Read the model definition and answer for the solid it produces. Units are mm, in the model's axes. Coordinates: 2 decimals unless noted, no trailing zeros. Order: outer loops, then holes, each group sorted by start corner. A loop starts at its lowest first (then second) coordinate and runs counter-clockwise, first axis right, second up. Notation, with made-up numbers: (28, 41.25) - (62, 41.25) arc R29 cw to (62, 65.25) - close; hole circle Ø4 at (-24.5, 75.25). An arc over 180 degrees is marked (long way). Write item = value, one per line.
from build123d import *

# Parameters (mm, degrees)
SKETCH1_W             = 80
SKETCH1_H             = 60
BOSS_EXTRUDE1_DEPTH   = 4.7625
M8_CLEARANCE_HOLE1_D  = 9
M6X1_0_TAPPED_HOLE2_D = 5
CHAMFER1_SIZE         = 1


with BuildPart() as part:
    # Sketch1 → Boss-Extrude1 (new, symmetric)
    with BuildSketch(Plane.XY):
        Rectangle(SKETCH1_W, SKETCH1_H)
    extrude(amount=BOSS_EXTRUDE1_DEPTH, both=True)

    # M8 Clearance Hole1 (through all)
    with Locations(Plane.XY.offset(4.7625)):
        with Locations((-30, 20), (30, 20), (30, -20), (-30, -20)):
            Hole(M8_CLEARANCE_HOLE1_D / 2)

    # M6x1.0 Tapped Hole2 (through all)
    with Locations(Plane.XY.offset(4.7625)):
        with Locations((-6.5, 23), (-6.5, -23)):
            Hole(M6X1_0_TAPPED_HOLE2_D / 2)

    # Chamfer1
    chamfer1_edges = [part.edges().sort_by_distance(p)[0] for p in [
        (-40, 30, 0),
        (40, 30, 0),
        (40, -30, 0),
        (-40, -30, 0),
    ]]
    chamfer(chamfer1_edges, length=CHAMFER1_SIZE)


solid = part.part
1) Determine the mould class of faces 1 (the face through (27.581, -16.206, -0.067)), 2 (the face through (-1, 30, 0)), 3 (the face through (-1, 0, 4.762)), 4 (the face through (-1, -30, 0)) for opening direction Y: pulls with the +Y half, pulls with the -Y half, needs draft (parallel to the pull), parting line crosses it, or undercut.
Returned:
face_1 = undercut
face_2 = pulls with the +Y half
face_3 = needs draft
face_4 = pulls with the -Y half
2) The part is cut by section B-B (z = 0.25). Determine the outline of the cut face in (x, y).
Returned:
outline = (-40, -29) - (-39, -30) - (39, -30) - (40, -29) - (40, 29) - (39, 30) - (-39, 30) - (-40, 29) - close; hole circle Ø9 at (-30, -20); hole circle Ø9 at (-30, 20); hole circle Ø5 at (-6.5, -23); hole circle Ø5 at (-6.5, 23); hole circle Ø9 at (30, -20); hole circle Ø9 at (30, 20)
3) The part is cut by section A-A (x = -30). Determine the outline of the cut face in (y, z).
Returned:
outline = (-30, -4.76) - (-24.5, -4.76) - (-24.5, 4.76) - (-30, 4.76) - close; (-15.5, -4.76) - (15.5, -4.76) - (15.5, 4.76) - (-15.5, 4.76) - close; (24.5, -4.76) - (30, -4.76) - (30, 4.76) - (24.5, 4.76) - close
4) Straight lines are drawn through the part: line 1 along Y through (x, z) = (-30, 0); line 2 along Y through (x, z) = (-6.5, -1.75); line 3 along X through (y, z) = (24, -1.5). For each, find the intervals that lie inside material, in ascending order. Write a range as from..to.
Returned:
line_1 = -30..-24.5, -15.5..15.5, 24.5..30
line_2 = -30..-25.5, -20.5..20.5, 25.5..30
line_3 = -40..-32.06, -27.94..-8.79, -4.21..27.94, 32.06..40
5) The part is cut by section C-C (y = -16.5). Determine the outline of the cut face in (x, z).
Returned:
outline = (-40, -4.76) - (-32.83, -4.76) - (-32.83, 4.76) - (-40, 4.76) - close; (-27.17, -4.76) - (27.17, -4.76) - (27.17, 4.76) - (-27.17, 4.76) - close; (32.83, -4.76) - (40, -4.76) - (40, 4.76) - (32.83, 4.76) - close
